Design review of the part built by this model. Coordinates are the model's own, in mm. A direction names the side the tool comes from. Coordinates: 2 decimals unless noted, no trailing zeros. Write each loop counter-clockwise with the first axis right and the second up, starting at its lowest first coordinate (ties: lowest second). Pieces come first, ordered by that corner, then holes. Notation, with made-up numbers: (61.5, -4.75) - (102.5, -4.75) arc R20 cw to (102.5, 0.25) - close; hole circle Ø9 at (-25.5, 78.5). An arc over 180 degrees is marked (long way). Answer as CSV lines item,"result". Start each with the question number.
Q1. Machinability: for faces 5 (the face through (2, 7.5, 9)), 6 (the face through (0, 12.5, 10)), which of the approach directions +Z, -Z, +X, -X, +Y, -Y give a long, thin tool a straight path to every point of the face, cutting with its end or side? Answer none if there is none.
Q2. We need section D-D (y = 10.5). Write out the cut boundary in (x, z).
Q3. Mouldability with a two-part tool opening along Z and no side actions: class faces 1 (the face through (2, 2.5, 8)), 2 (the face through (0, 0, 20)), 3 (the face through (-7, 0, 18)), 4 (the face through (0, 0, 0)) as pulls with the +Z half, pulls with the -Z half, needs draft (parallel to the pull), parting line crosses it, or undercut.
Q4. We need section C-C (x = 0). Write out the cut boundary in (y, z), plus the area to 3 significant figures.
Q5. We need section B-B (z = 17). Write out the cut boundary in (x, y), plus the area to 3 significant figures.
Q6. For line 1 along X through (y, z) = (-0.35, 17); line 2 along Y through (x, z) = (7.5, 4.75); line 3 along X through (y, z) = (9, 11.25), list the stretches that pass through material, from the lowest coordinate up. Write a range as [from, to].
Q7. We need section A-A (x = 7). Write out the cut boundary in (y, z).
Q8. Clearance check with flat-ended pins moving along their axes: pin 1 (3 mm diameter, centred on x = 7, z = 3, fed in from +Y); pin 2 (5 mm diameter, centred on x = -4, z = 12.5, fed in from +Y). State where each tip first meets the part, or that it passes through.
from build123d import *

# Parameters (mm, degrees)
SKETCH1_W           = 20
SKETCH1_H           = 5
BOSS_EXTRUDE1_DEPTH = 20
SKETCH2_R           = 2.5
BOSS_EXTRUDE2_DEPTH = 10
SKETCH3_R           = 1
CUT_EXTRUDE1_DEPTH  = 25.494897428
CUT_EXTRUDE2_START  = -5
SKETCH4_R           = 2.5
SKETCH4_R_2         = 2
CUT_EXTRUDE2_DEPTH  = 5


with BuildPart() as part:
    # Sketch1 → Boss-Extrude1 (new body)
    with BuildSketch(Plane.XY):
        Rectangle(SKETCH1_W, SKETCH1_H)
    extrude(amount=BOSS_EXTRUDE1_DEPTH)

    # Sketch2 → Boss-Extrude2 (add)
    with BuildSketch(Plane(origin=(0, 2.5, 0), x_dir=(1, 0, 0), z_dir=(0, 1, 0))):
        with Locations(Location((0, -10, 0), (0, 0, 270))):
            Circle(SKETCH2_R)
    extrude(amount=BOSS_EXTRUDE2_DEPTH)

    # Sketch3 → Cut-Extrude1 (cut, through all)
    with BuildSketch(Plane(origin=(0, 2.5, 0), x_dir=(1, 0, 0), z_dir=(0, 1, 0))):
        with Locations(Location((-7, -3, 0), (0, 0, 270))):
            Circle(SKETCH3_R)
        with Locations(Location((7, -3, 0), (0, 0, 270))):
            Circle(SKETCH3_R)
        with Locations(Location((-7, -17, 0), (0, 0, 270))):
            Circle(SKETCH3_R)
        with Locations(Location((7, -17, 0), (0, 0, 270))):
            Circle(SKETCH3_R)
    extrude(amount=-CUT_EXTRUDE1_DEPTH, mode=Mode.SUBTRACT)

    # Sketch4 → Cut-Extrude2 (cut)
    with BuildSketch(Plane(origin=(0, 12.5, 0), x_dir=(1, 0, 0), z_dir=(0, 1, 0)).offset(CUT_EXTRUDE2_START)):
        with Locations(Location((0, -10, 0), (0, 0, 270))):
            Circle(SKETCH4_R)
        with Locations(Location((0, -10, 0), (0, 0, 270))):
            Circle(SKETCH4_R_2, mode=Mode.SUBTRACT)
    extrude(amount=CUT_EXTRUDE2_DEPTH, mode=Mode.SUBTRACT)


solid = part.part
Results list:
1,face 5,"+Y"
1,face 6,"+Z, -Z, +X, -X, +Y"
2,outline,"circle Ø4 at (0, 10)"
3,face 1,"needs draft"
3,face 2,"pulls with the +Z half"
3,face 3,"undercut"
3,face 4,"pulls with the -Z half"
4,outline,"(-2.5, 0) - (2.5, 0) - (2.5, 7.5) - (7.5, 7.5) - (7.5, 8) - (12.5, 8) - (12.5, 12) - (7.5, 12) - (7.5, 12.5) - (2.5, 12.5) - (2.5, 20) - (-2.5, 20) - close"
4,area,"145 mm2"
5,outline,"(-10, -2.5) - (-8, -2.5) - (-8, 2.5) - (-10, 2.5) - close; (-6, -2.5) - (6, -2.5) - (6, 2.5) - (-6, 2.5) - close; (8, -2.5) - (10, -2.5) - (10, 2.5) - (8, 2.5) - close"
5,area,"80.0 mm2"
6,line 1,"x = [-10, -8], [-6, 6], [8, 10]"
6,line 2,"y = [-2.5, 2.5]"
6,line 3,"x = [-1.56, 1.56]"
7,outline,"(-2.5, 0) - (2.5, 0) - (2.5, 2) - (-2.5, 2) - close; (-2.5, 4) - (2.5, 4) - (2.5, 16) - (-2.5, 16) - close; (-2.5, 18) - (2.5, 18) - (2.5, 20) - (-2.5, 20) - close"
8,pin 1,"stops at y = 2.5"
8,pin 2,"stops at y = 7.5"
